Can you work these out from the model? Positions are in its coordinate system, mm. Face numbers are marked on the shaded views. A direction names the side the tool comes from. Coordinates: 2 decimals unless noted, no trailing zeros. Loops run counter-clockwise (first coordinate to the right, second up) from the corner with the lowest first, then second, coordinate; pieces in that order, holes last.
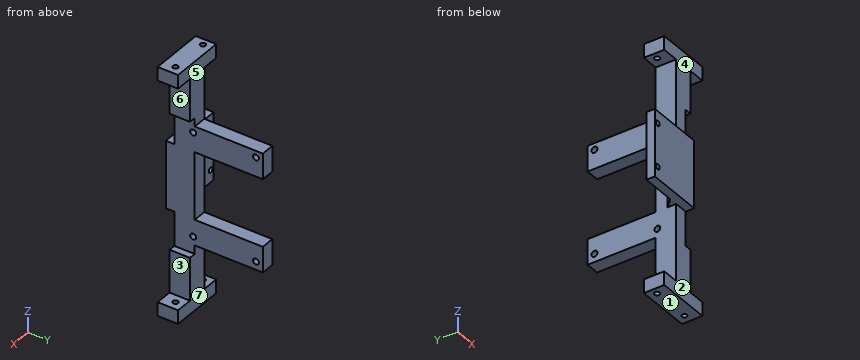
```python
from build123d import *

# Parameters (mm, degrees)
SKETCH_1_W          = 12
SKETCH_1_H          = 12
EXTRUDE_1_DEPTH     = 129.5
SKETCH_3_W          = 32
SKETCH_3_H          = 12
EXTRUDE_2_DEPTH     = 8
SKETCH_4_W          = 32
SKETCH_4_H          = 12
EXTRUDE_3_DEPTH     = 8
SKETCH_5_W          = 79.5
SKETCH_5_H          = 52
EXTRUDE_4_DEPTH     = 8
SKETCH_6_W          = 59.5
SKETCH_6_H          = 40
CUT_EXTRUDE_1_DEPTH = 10
SKETCH_10_W         = 8
SKETCH_10_H         = 40
EXTRUDE_7_DEPTH     = 10
SKETCH_11_W         = 8
SKETCH_11_H         = 40
EXTRUDE_8_DEPTH     = 10
SKETCH_13_W         = 8
SKETCH_13_H         = 40
CUT_EXTRUDE_3_DEPTH = 5
SKETCH_14_W         = 8
SKETCH_14_H         = 40
CUT_EXTRUDE_4_DEPTH = 5
SKETCH_17_R         = 1.55
CUT_EXTRUDE_5_DEPTH = 146.870661889
SKETCH_17_2_R       = 1.55
CUT_EXTRUDE_6_DEPTH = 146.870661889
SKETCH_19_W         = 4
SKETCH_19_H         = 79.5
CUT_EXTRUDE_7_DEPTH = 145.091117006
SKETCH_20_W         = 8
SKETCH_20_H         = 39.5
EXTRUDE_9_DEPTH     = 5
SKETCH_21_W         = 39.5
SKETCH_21_H         = 5
EXTRUDE_10_DEPTH    = 25
SKETCH_23_R         = 1.55
CUT_EXTRUDE_8_DEPTH = 153.040290713
CUT_EXTRUDE_9_REACH = 150.699
SKETCH_25_R         = 1.75
SKETCH_25_R_2       = 1.726022487
EXTRUDE_11_DEPTH    = 39.5


with BuildPart() as part:
    # 草图1 → 凸台-拉伸1 (new body)
    with BuildSketch(Plane.XY):
        Rectangle(SKETCH_1_W, SKETCH_1_H)
    extrude(amount=EXTRUDE_1_DEPTH)

    # 草图3 → 凸台-拉伸2 (add)
    with BuildSketch(Plane.XY.offset(129.5)):
        Rectangle(SKETCH_3_W, SKETCH_3_H)
    extrude(amount=EXTRUDE_2_DEPTH)

    # 草图4 → 凸台-拉伸3 (add)
    with BuildSketch(Plane(origin=(0, 0, 0), x_dir=(-1, 0, 0), z_dir=(0, 0, -1))):
        Rectangle(SKETCH_4_W, SKETCH_4_H)
    extrude(amount=EXTRUDE_3_DEPTH)

    # 草图5 → 凸台-拉伸4 (add)
    with BuildSketch(Plane.ZY.offset(6)):
        with Locations((64.75, 20)):
            Rectangle(SKETCH_5_W, SKETCH_5_H)
    extrude(amount=-EXTRUDE_4_DEPTH)

    # 草图6 → 切除-拉伸1 (cut)
    with BuildSketch(Plane(origin=(2, 0, 0), x_dir=(0, 0, -1), z_dir=(1, 0, 0))):
        with Locations((-64.75, 26)):
            Rectangle(SKETCH_6_W, SKETCH_6_H)
    extrude(amount=-CUT_EXTRUDE_1_DEPTH, mode=Mode.SUBTRACT)

    # 草图10 → 凸台-拉伸7 (add)
    with BuildSketch(Plane.XY.offset(35)):
        with Locations((-2, 26)):
            Rectangle(SKETCH_10_W, SKETCH_10_H)
    extrude(amount=EXTRUDE_7_DEPTH)

    # 草图11 → 凸台-拉伸8 (add)
    with BuildSketch(Plane(origin=(0, 0, 94.5), x_dir=(-1, 0, 0), z_dir=(0, 0, -1))):
        with Locations((2, 26)):
            Rectangle(SKETCH_11_W, SKETCH_11_H)
    extrude(amount=EXTRUDE_8_DEPTH)

    # 草图13 → 切除-拉伸3 (cut)
    with BuildSketch(Plane(origin=(0, 0, 25), x_dir=(-1, 0, 0), z_dir=(0, 0, -1))):
        with Locations((2, 26)):
            Rectangle(SKETCH_13_W, SKETCH_13_H)
    extrude(amount=-CUT_EXTRUDE_3_DEPTH, mode=Mode.SUBTRACT)

    # 草图14 → 切除-拉伸4 (cut)
    with BuildSketch(Plane.XY.offset(104.5)):
        with Locations((-2, 26)):
            Rectangle(SKETCH_14_W, SKETCH_14_H)
    extrude(amount=-CUT_EXTRUDE_4_DEPTH, mode=Mode.SUBTRACT)

    # 草图17 → 切除-拉伸5 (cut, through all)
    with BuildSketch(Plane(origin=(0, 0, 129.5), x_dir=(-1, 0, 0), z_dir=(0, 0, -1))):
        with Locations((12, 1)):
            Circle(SKETCH_17_R)
        with Locations((-11, 1)):
            Circle(SKETCH_17_R)
    extrude(amount=-CUT_EXTRUDE_5_DEPTH, mode=Mode.SUBTRACT)

    # 草图17<2> → 切除-拉伸6 (cut, through all)
    with BuildSketch(Plane(origin=(0, 0, 129.5), x_dir=(-1, 0, 0), z_dir=(0, 0, -1))):
        with Locations((12, 1)):
            Circle(SKETCH_17_2_R)
        with Locations((-11, 1)):
            Circle(SKETCH_17_2_R)
    extrude(amount=CUT_EXTRUDE_6_DEPTH, mode=Mode.SUBTRACT)

    # 草图19 → 切除-拉伸7 (cut, through all)
    with BuildSketch(Plane(origin=(0, 6, 0), x_dir=(1, 0, 0), z_dir=(0, 1, 0))):
        with Locations((4, -64.75)):
            Rectangle(SKETCH_19_W, SKETCH_19_H)
    extrude(amount=-CUT_EXTRUDE_7_DEPTH, mode=Mode.SUBTRACT)

    # 草图20 → 凸台-拉伸9 (add)
    with BuildSketch(Plane.XZ.offset(6)):
        with Locations((-2, 64.75)):
            Rectangle(SKETCH_20_W, SKETCH_20_H)
    extrude(amount=EXTRUDE_9_DEPTH)

    # 草图21 → 凸台-拉伸10 (add)
    with BuildSketch(Plane.ZY.offset(6)):
        with Locations((64.75, -8.5)):
            Rectangle(SKETCH_21_W, SKETCH_21_H)
    extrude(amount=EXTRUDE_10_DEPTH)

    # 草图23 → 切除-拉伸8 (cut, through all)
    with BuildSketch(Plane.XZ.offset(11)):
        with Locations(Location((-28.5, 77.45, 0), (0, 0, 270))):
            Circle(SKETCH_23_R)
        with Locations(Location((-28.5, 52.05, 0), (0, 0, 270))):
            Circle(SKETCH_23_R)
    extrude(amount=-CUT_EXTRUDE_8_DEPTH, mode=Mode.SUBTRACT)

    # 草图25 → 切除-拉伸9 (cut, up to next)
    with BuildSketch(Plane(origin=(2, 0, 0), x_dir=(0, 0, -1), z_dir=(1, 0, 0)), mode=Mode.PRIVATE) as cut_extrude_9_sk1:
        with Locations((-95.65, 41.95)):
            Circle(SKETCH_25_R)
    cut_extrude_9_tool1 = extrude(cut_extrude_9_sk1.sketch, amount=-CUT_EXTRUDE_9_REACH, mode=Mode.PRIVATE) & part.part
    # 草图25 → 切除-拉伸9 (cut, up to next)
    with BuildSketch(Plane(origin=(2, 0, 0), x_dir=(0, 0, -1), z_dir=(1, 0, 0)), mode=Mode.PRIVATE) as cut_extrude_9_sk2:
        with Locations((-95.65, 5.05)):
            Circle(SKETCH_25_R)
    cut_extrude_9_tool2 = extrude(cut_extrude_9_sk2.sketch, amount=-CUT_EXTRUDE_9_REACH, mode=Mode.PRIVATE) & part.part
    # 草图25 → 切除-拉伸9 (cut, up to next)
    with BuildSketch(Plane(origin=(2, 0, 0), x_dir=(0, 0, -1), z_dir=(1, 0, 0)), mode=Mode.PRIVATE) as cut_extrude_9_sk3:
        with Locations((-34.826022487, 5.05)):
            Circle(SKETCH_25_R_2)
    cut_extrude_9_tool3 = extrude(cut_extrude_9_sk3.sketch, amount=-CUT_EXTRUDE_9_REACH, mode=Mode.PRIVATE) & part.part
    # 草图25 → 切除-拉伸9 (cut, up to next)
    with BuildSketch(Plane(origin=(2, 0, 0), x_dir=(0, 0, -1), z_dir=(1, 0, 0)), mode=Mode.PRIVATE) as cut_extrude_9_sk4:
        with Locations((-34.85, 41.95)):
            Circle(SKETCH_25_R)
    cut_extrude_9_tool4 = extrude(cut_extrude_9_sk4.sketch, amount=-CUT_EXTRUDE_9_REACH, mode=Mode.PRIVATE) & part.part
    add(cut_extrude_9_tool1.solids().sort_by_distance((2, 41.95, 95.65))[0], mode=Mode.SUBTRACT)
    add(cut_extrude_9_tool2.solids().sort_by_distance((2, 5.05, 95.65))[0], mode=Mode.SUBTRACT)
    add(cut_extrude_9_tool3.solids().sort_by_distance((2, 5.05, 34.826022))[0], mode=Mode.SUBTRACT)
    add(cut_extrude_9_tool4.solids().sort_by_distance((2, 41.95, 34.85))[0], mode=Mode.SUBTRACT)

    # 草图26 → 凸台-拉伸11 (add)
    with BuildSketch(Plane(origin=(0, 0, 45), x_dir=(-1, 0, 0), z_dir=(0, 0, -1))):
        Polygon((6, -6), (6, -1), (11, -6), align=None)
    extrude(amount=-EXTRUDE_11_DEPTH)


solid = part.part
```
Item 1: We'd pull the mould along Z, two halves only. Please class the marked faces 1, 2 and 3: +Z half, -Z half, draft (parallel to the pull), parting line (faces both ways), or undercut.
Results are:
face 1: -Z half
face 2: draft
face 3: undercut
Item 2: On a 3-axis mill with a long thin cutter (end or side, diameter ignored), from which of +Z, -Z, +X, -X, +Y, -Y can I reach the whole of each face in a straight line? I mean the marked faces 4, 5, 6 and 7. Say none if no direction works.
Results are:
face 4: +Z, +X, -X, -Y
face 5: +Z, +X, -X, +Y
face 6: +X, +Y, -Y
face 7: -Z, +X, -X, +Y
Item 3: Suppose I cut it at A-A, the plane x = 11. Please give me the cut outline in (y, z), plus the area to 3 significant figures.
Results are:
outline: (-6, -8) - (-0.55, -8) - (-0.55, 0) - (-6, 0) - close; (-6, 129.5) - (-0.55, 129.5) - (-0.55, 137.5) - (-6, 137.5) - close; (2.55, -8) - (6, -8) - (6, 0) - (2.55, 0) - close; (2.55, 129.5) - (6, 129.5) - (6, 137.5) - (2.55, 137.5) - close
area: 142 mm2
Item 4: I need wall thicknesses on line 1 along Y through (x, z) = (-3.25, 95.65); line 2 along X through (y, z) = (1, -4.5); line 3 along Y through (x, z) = (11, 133). Which ranges of each line are inside material? Lowest first, please.
Results are:
line 1: y = -6 to 3.3, 6.8 to 40.2, 43.7 to 46
line 2: x = -16 to -13.55, -10.45 to 9.45, 12.55 to 16
line 3: y = -6 to -0.55, 2.55 to 6
Item 5: I'm going to push flat-ended pins straight in: P1, Ø6.5, axis at x = -2, y = 23.5, coming from the +Z side; P2, Ø3, axis at y = 41.95, z = 95.65, coming from the -X side; P3, Ø8, axis at x = 5.5, y = 27, coming from the -Z side; P4, Ø4, axis at y = -1.5, z = -4.5, coming from the -X side. Where does each tip first touch, or does it pass through?
Results are:
P1: stops at z = 99.5
P2: passes through
P3: stops at z = 30
P4: stops at x = -16
Item 6: Suppose I cut it at D-D, the plane y = 1. Count the separate pieces of the cut face and the enclosed holes in it, plus the area to 3 significant figures.
Results are:
separate pieces: 5
enclosed holes: 0
area: 1,650 mm2
Item 7: Suppose I cut it at C-C, the plane z = 77.45. Please give me the cut outline in (x, y).
Results are:
outline: (-31, -11) - (-30.05, -11) - (-30.05, -6) - (-31, -6) - close; (-26.95, -11) - (2, -11) - (2, 6) - (-6, 6) - (-6, -1) - (-11, -6) - (-26.95, -6) - close
Item 8: Suppose I cut it at B-B, the plane y = 14.5. Please give me the cut outline in (x, z), plus the area to 3 significant figures.
Results are:
outline: (-6, 30) - (2, 30) - (2, 45) - (-6, 45) - close; (-6, 84.5) - (2, 84.5) - (2, 99.5) - (-6, 99.5) - close
area: 240 mm2
